Can you work these out from the model? Positions are in its coordinate system, mm. A direction names the side the tool comes from. Give positions to 0.01 mm unless a question says otherwise; leave off trailing zeros. Order: outer loops, then holes, each group sorted by start corner. A loop starts at its lowest first (then second) coordinate and runs counter-clockwise, first axis right, second up. Notation, with made-up numbers: M 55,-31 L 107,-31 A22 ccw 107,-17 Z; hole C 17,62.5 d5. An arc over 180 degrees is marked long. Write each question's results on one line, items separated by ' | '.
from build123d import *

# Parameters (mm, degrees)
BOSS_EXTRUDE1_DEPTH = 34.2
SKETCH4_R           = 2
SKETCH4_R_2         = 1
CUT_EXTRUDE3_DEPTH  = 7
FILLET1_R           = 3
SKETCH5_R           = 10
CUT_EXTRUDE4_DEPTH  = 5
SKETCH6_R           = 3
SKETCH6_R_2         = 1.5
CUT_EXTRUDE5_DEPTH  = 5


with BuildPart() as part:
    # Sketch1 → Boss-Extrude1 (new body)
    with BuildSketch(Plane(origin=(0, 0, 0), x_dir=(1, 0, 0), z_dir=(0, 1, 0))):
        Polygon((0, 0), (58, 0), (58, 47), (63, 47), (63, -2), (60, -7), (58, -7), (0, -7), (-2, -7), (-5, -2), (-5, 47), (0, 47), align=None)
    extrude(amount=BOSS_EXTRUDE1_DEPTH)

    # Sketch4 → Cut-Extrude3 (cut)
    with BuildSketch(Plane(origin=(0, 0, 0), x_dir=(-1, 0, 0), z_dir=(0, 0, -1))):
        with Locations((-29, 24.6)):
            Circle(SKETCH4_R)
        with Locations((-36.5, 17.1)):
            Circle(SKETCH4_R)
        with Locations((-21.5, 17.1)):
            Circle(SKETCH4_R)
        with Locations((-29, 9.6)):
            Circle(SKETCH4_R)
        with Locations((-29, 17.1)):
            Circle(SKETCH4_R_2)
    extrude(amount=-CUT_EXTRUDE3_DEPTH, mode=Mode.SUBTRACT)

    # Fillet1
    fillet1_edges = [part.edges().sort_by_distance(p)[0] for p in [
        (60.5, 0, -47),
        (-2.5, 0, -47),
        (60.5, 34.2, -47),
        (-2.5, 34.2, -47),
    ]]
    fillet(fillet1_edges, radius=FILLET1_R)

    # Sketch5 → Cut-Extrude4 (cut)
    with BuildSketch(Plane.ZY.offset(5)):
        with Locations((-27, 17.1)):
            Circle(SKETCH5_R)
    extrude(amount=-CUT_EXTRUDE4_DEPTH, mode=Mode.SUBTRACT)

    # Sketch6 → Cut-Extrude5 (cut)
    with BuildSketch(Plane(origin=(63, 0, 0), x_dir=(0, 0, -1), z_dir=(1, 0, 0))):
        with Locations((27, 17.1)):
            Circle(SKETCH6_R)
        with Locations((27, 27.1)):
            Circle(SKETCH6_R_2)
        with Locations((37, 17.1)):
            Circle(SKETCH6_R_2)
        with Locations((27, 7.1)):
            Circle(SKETCH6_R_2)
        with Locations((17, 17.1)):
            Circle(SKETCH6_R_2)
    extrude(amount=-CUT_EXTRUDE5_DEPTH, mode=Mode.SUBTRACT)


solid = part.part
(1) Imagine slicing it at D-D, the plane y = 29.5. Write out the boundary of the cut face in (x, z), plus the area to 3 significant figures.
Data:
outline: M -5,-47 L 0,-47 L 0,0 L 58,0 L 58,-47 L 63,-47 L 63,2 L 60,7 L -2,7 L -5,2 Z | area: 931 mm2
(2) I need wall thicknesses on L1, parallel to Y at x = 29, z = 4.25; L2, parallel to Y at x = 59.7, z = -27; L3, parallel to X at y = 5.5, z = -7. Which ranges of each line are inside material? Lowest first, please. Write a range as from..to.
Data:
L1: y = 0..7.6, 11.6..16.1, 18.1..22.6, 26.6..34.2 | L2: y = 0..5.6, 8.6..14.1, 20.1..25.6, 28.6..34.2 | L3: x = -5..0, 58..63
(3) Imagine slicing it at A-A, the plane z = -9.5. Write out the boundary of the cut face in (x, y), plus the area to 3 significant figures.
Data:
outline: M -5,0 L 0,0 L 0,34.2 L -5,34.2 Z; M 58,0 L 63,0 L 63,34.2 L 58,34.2 Z | area: 342 mm2
(4) Imagine slicing it at B-B, the plane x = 36.5. Write out the boundary of the cut face in (y, z).
Data:
outline: M 0,0 L 15.1,0 L 15.1,7 L 0,7 Z; M 19.1,0 L 34.2,0 L 34.2,7 L 19.1,7 Z
(5) Will these pins go through, and if not, where does the flat tip stop? P1, Ø18, axis at y = 17.1, z = -27, coming from the +X side; P2, Ø6.5, axis at x = 21.5, y = 17.1, coming from the -Z side; P3, Ø2.5, axis at y = 7.1, z = -27, coming from the +X side.
Data:
P1: stops at x = 63 | P2: stops at z = 0 | P3: stops at x = 0
(6) For faces 1 (the face through (-2.535, 13.27, -17.763)), 2 (the face through (0, 24, -19)), 3 (the face through (29, 21, 7)), which set-ups out of +Z, -Z, +X, -X, +Y, -Y let a thin tool reach every point of the face, with its end or its side?
Data:
face 1: -X | face 2: -Z, +Y, -Y | face 3: +Z, +X, -X, +Y, -Y
(7) Imagine slicing it at C-C, the plane z = -21. Write out the boundary of the cut face in (x, y).
Data:
outline: M -5,0 L 0,0 L 0,9.1 L -5,9.1 Z; M -5,25.1 L 0,25.1 L 0,34.2 L -5,34.2 Z; M 58,0 L 63,0 L 63,34.2 L 58,34.2 Z
(8) We'd pull the mould along Y, two halves only. Please class faces 4 (the face through (60.54, 33.34, -46.1)), 5 (the face through (60.54, 18.11, -35.89)), 6 (the face through (60.54, 0.86, -46.1)), 7 (the face through (60.54, 27.17, -25.5)): +Y half, -Y half, draft (parallel to the pull), parting line (faces both ways), or undercut.
Data:
face 4: +Y half | face 5: undercut | face 6: -Y half | face 7: undercut
